Solid Edge part; units mm, degrees
sketch "Sketch1" plane through (0, 0, 0) normal (0, 0, 1) x (1, 0, 0)
  line L0 (0, 54.5388) -> (13, 54.5388)
  line L1 (13, 54.5388) -> (13, -45.4612)
  line L2 (13, -45.4612) -> (0, -45.4612)
  line L3 (0, -45.4612) -> (0, -42.4612)
  line L4 (0, -42.4612) -> (11, -42.4612)
  line L5 (11, -42.4612) -> (11, 51.5388)
  line L6 (11, 51.5388) -> (0, 51.5388)
  line L7 (0, 51.5388) -> (0, 54.5388)
  dimension "D1" = 13
  dimension "D2" = 13
extrude "Protrusion1" add sketch "Sketch1" along normal mid plane 55
sketch "Sketch2" plane through (13, 4.5388, 0) normal (1, 0, 0) x (0, 1, 0)
  line L0 (-50, -6.5) -> (50, -6.5)
  line L1 (50, -6.5) -> (50, -3.5)
  line L2 (50, -3.5) -> (-50, -3.5)
  line L3 (-50, -3.5) -> (-50, -6.5)
  dimension "D1" = 50
  dimension "D2" = 50
extrude "ExtrudedProtrusion_3" add sketch "Sketch2" along normal blind 25
sketch "Sketch3" plane through (10.5, 4.5388, 27.5) normal (0, 0, 1) x (1, 0, 0)
  line L0 (-10.5, 47) -> (0.5, 47)
  line L1 (0.5, 47) -> (0.5, 50)
  line L2 (0.5, 50) -> (-10.5, 50)
  line L3 (-10.5, 50) -> (-10.5, 47)
extrude "ExtrudedCutout_1" cut sketch "Sketch3" against normal blind 45
properties material "ABS Plastic, high impact"
Verification items for the finished model (mm, model axes). A direction names the side the tool comes from. Coordinates: 2 decimals unless noted, no trailing zeros. Order: outer loops, then holes, each group sorted by start corner. A loop starts at its lowest first (then second) coordinate and runs counter-clockwise, first axis right, second up. Notation, with made-up numbers: (1, -33) -> (33, -33) arc R27 cw to (33, -2) -> close; hole circle Ø7 at (32, -9.5). An arc over 180 degrees is marked (long way). Answer as CSV lines item,"result". Start each with the question number.
1) Cross-section at A-A, the plane x = 6. Record the boundary of the cut face in (y, z).
2) Release check for a two-part mould opening along Y. For faces 1 (the face through (5, -42.461, 0)), 2 (the face through (11, -45.461, 0)), 3 (the face through (11, 5, 0)), 4 (the face through (5, 53, -17.5)) record: released by +Y, released by -Y, zero draft, split by the parting line, or undercut.
3) Set-up check for faces 5 (the face through (12, -6, 27.5)), 6 (the face through (6, 51.539, -23)), 7 (the face through (25, 5, -3.5)), 8 (the face through (13, 5, -17)), 9 (the face through (12, 54.539, -10)): record each of +Z, -Z, +X, -X, +Y, -Y from which the full face is reachable in a straight line by a thin tool's end or side.
4) Gauge pin test, flat ends, axial feed: pin 1 Ø20 at (x, y) = (26, -14.5) entering from +Z; pin 2 Ø4 at (y, z) = (37, -0.5) entering from -X; pin 3 Ø4 at (x, z) = (5, 19) entering from +Y. Record the tip position at first contact, or that the pin passes through.
5) Material ranges on L1, parallel to Y at x = 9, z = 10; L2, parallel to X at y = -30, z = -6; L3, parallel to X at y = -22, z = -11.5, recorded low to high. Write a range as [from, to].
6) Cross-section at D-D, the plane x = 23. Record the boundary of the cut face in (y, z), then the cut area to 3 significant figures.
7) Cross-section at C-C, the plane y = 9. Record the boundary of the cut face in (x, z), then the cut area to 3 significant figures.
8) Cross-section at B-B, the plane z = -21. Record the boundary of the cut face in (x, y), then the cut area to 3 significant figures.
Conclusion:
1,outline,"(-45.46, -27.5) -> (-42.46, -27.5) -> (-42.46, 27.5) -> (-45.46, 27.5) -> close; (51.54, -27.5) -> (54.54, -27.5) -> (54.54, -17.5) -> (51.54, -17.5) -> close"
2,face 1,"undercut"
2,face 2,"released by -Y"
2,face 3,"undercut"
2,face 4,"zero draft"
3,face 5,"+Z, +X, -X, +Y, -Y"
3,face 6,"+Z, -Z, -X"
3,face 7,"+Z, +X, +Y, -Y"
3,face 8,"-Z, +X, +Y, -Y"
3,face 9,"+Z, -Z, +X, -X, +Y"
4,pin 1,"stops at z = -3.5"
4,pin 2,"stops at x = 11"
4,pin 3,"stops at y = -42.46"
5,L1,"y = [-45.46, -42.46]"
5,L2,"x = [11, 38]"
5,L3,"x = [11, 13]"
6,outline,"(-45.46, -6.5) -> (54.54, -6.5) -> (54.54, -3.5) -> (-45.46, -3.5) -> close"
6,area,"300 mm²"
7,outline,"(11, -27.5) -> (13, -27.5) -> (13, -6.5) -> (38, -6.5) -> (38, -3.5) -> (13, -3.5) -> (13, 27.5) -> (11, 27.5) -> close"
7,area,"185 mm²"
8,outline,"(0, -45.46) -> (13, -45.46) -> (13, 54.54) -> (0, 54.54) -> (0, 51.54) -> (11, 51.54) -> (11, -42.46) -> (0, -42.46) -> close"
8,area,"266 mm²"
